```python
from build123d import *

# Parameters (mm, degrees)
SKETCH1_W           = 300
SKETCH1_H           = 80
BOSS_EXTRUDE1_DEPTH = 7
CHAMFER1_SIZE       = 15
CHAMFER1_SIZE2      = 25.980762114
CHAMFER3_SIZE       = 15
CHAMFER3_SIZE2      = 25.980762114
SKETCH2_R           = 11
CUT_EXTRUDE1_DEPTH  = 10
SKETCH3_R           = 11
SKETCH3_R_2         = 9.5
BOSS_EXTRUDE3_DEPTH = 0.8
CUT_EXTRUDE2_DEPTH  = 8
SKETCH5_R           = 15
CUT_EXTRUDE3_DEPTH  = 8
CUT_EXTRUDE4_DEPTH  = 8
SKETCH7_R           = 8
CUT_EXTRUDE6_DEPTH  = 8
SKETCH8_R           = 8
SKETCH8_R_2         = 7
BOSS_EXTRUDE4_DEPTH = 1.8
SKETCH9_R           = 1.5
CUT_EXTRUDE7_DEPTH  = 8
SKETCH10_R          = 12
CUT_EXTRUDE8_DEPTH  = 1
SKETCH11_R          = 1.5
CUT_EXTRUDE9_DEPTH  = 8
SKETCH12_R          = 2.6
SKETCH12_R_2        = 2.5
CUT_EXTRUDE10_DEPTH = 8
SKETCH13_R          = 4
CUT_EXTRUDE11_DEPTH = 4
SKETCH14_R          = 1.75
CUT_EXTRUDE12_DEPTH = 8
CUT_EXTRUDE13_DEPTH = 8
CUT_EXTRUDE14_DEPTH = 8
CUT_EXTRUDE15_DEPTH = 8
SKETCH18_R          = 3.25
CUT_EXTRUDE16_DEPTH = 4
CHAMFER4_SIZE       = 2
FILLET1_R           = 3
FILLET2_R           = 3
SKETCH19_R          = 2.6
CUT_EXTRUDE17_DEPTH = 8
SKETCH20_R          = 4.5
CUT_EXTRUDE18_DEPTH = 5
SKETCH21_W          = 9
SKETCH21_H          = 5
CUT_EXTRUDE19_DEPTH = 5
CHAMFER5_SIZE       = 5


with BuildPart() as part:
    # Sketch1 → Boss-Extrude1 (new body)
    with BuildSketch(Plane.XY):
        with Locations((150, 40)):
            Rectangle(SKETCH1_W, SKETCH1_H)
    extrude(amount=BOSS_EXTRUDE1_DEPTH)

    # Chamfer1
    chamfer1_edges = [part.edges().sort_by_distance(p)[0] for p in [
        (0, 0, 3.5),
    ]]
    chamfer1_side = [part.faces().sort_by_distance(p)[0] for p in [
        (0, 40, 3.5),
    ]]
    chamfer(chamfer1_edges, length=CHAMFER1_SIZE, length2=CHAMFER1_SIZE2, reference=chamfer1_side[0])

    # Chamfer3
    chamfer3_edges = [part.edges().sort_by_distance(p)[0] for p in [
        (0, 80, 3.5),
    ]]
    chamfer3_side = [part.faces().sort_by_distance(p)[0] for p in [
        (0, 47.5, 3.5),
    ]]
    chamfer(chamfer3_edges, length=CHAMFER3_SIZE, length2=CHAMFER3_SIZE2, reference=chamfer3_side[0])

    # Sketch2 → Cut-Extrude1 (cut)
    with BuildSketch(Plane.XY.offset(7)):
        with Locations((35, 40)):
            Circle(SKETCH2_R)
    extrude(amount=-CUT_EXTRUDE1_DEPTH, mode=Mode.SUBTRACT)

    # Sketch3 → Boss-Extrude3 (add)
    with BuildSketch(Plane.XY.offset(7)):
        with Locations((35, 40)):
            Circle(SKETCH3_R)
        with Locations((35, 40)):
            Circle(SKETCH3_R_2, mode=Mode.SUBTRACT)
    extrude(amount=-BOSS_EXTRUDE3_DEPTH)

    # Sketch4 → Cut-Extrude2 (cut, through all)
    with BuildSketch(Plane.XY.offset(7)):
        with BuildLine():
            Line((163.324941262, 70), (163.324941262, 40))
            ThreePointArc((163.324941262, 40), (162.324941262, 39), (161.324941262, 40))
            Line((161.324941262, 40), (161.324941262, 70))
            ThreePointArc((161.324941262, 70), (162.324941262, 71), (163.324941262, 70))
        make_face()
    extrude(amount=-CUT_EXTRUDE2_DEPTH, mode=Mode.SUBTRACT)

    # Sketch5 → Cut-Extrude3 (cut, through all)
    with BuildSketch(Plane.XY.offset(7)):
        with Locations((250, 40)):
            Circle(SKETCH5_R)
    extrude(amount=-CUT_EXTRUDE3_DEPTH, mode=Mode.SUBTRACT)

    # Sketch6 → Cut-Extrude4 (cut)
    with BuildSketch(Plane(origin=(0, 0, 0), x_dir=(-1, 0, 0), z_dir=(0, 0, -1))):
        with BuildLine():
            Line((-158.324941262, 70), (-158.324941262, 40))
            ThreePointArc((-158.324941262, 40), (-162.324941262, 36), (-166.324941262, 40))
            Line((-166.324941262, 40), (-166.324941262, 70))
            ThreePointArc((-166.324941262, 70), (-162.324941262, 74), (-158.324941262, 70))
        make_face()
    extrude(amount=-CUT_EXTRUDE4_DEPTH, mode=Mode.SUBTRACT)

    # Sketch7 → Cut-Extrude6 (cut, through all)
    with BuildSketch(Plane.XY.offset(7)):
        with Locations((113.691629607, 65)):
            Circle(SKETCH7_R)
    extrude(amount=-CUT_EXTRUDE6_DEPTH, mode=Mode.SUBTRACT)

    # Sketch8 → Boss-Extrude4 (add)
    with BuildSketch(Plane.XY.offset(7)):
        with Locations((113.691629607, 65)):
            Circle(SKETCH8_R)
        with Locations((113.691629607, 65)):
            Circle(SKETCH8_R_2, mode=Mode.SUBTRACT)
    extrude(amount=-BOSS_EXTRUDE4_DEPTH)

    # Sketch9 → Cut-Extrude7 (cut, through all)
    with BuildSketch(Plane(origin=(0, 0, 0), x_dir=(-1, 0, 0), z_dir=(0, 0, -1))):
        with Locations((-113.691629607, 74.75)):
            Circle(SKETCH9_R)
        with Locations((-105.24788192, 69.875)):
            Circle(SKETCH9_R)
        with Locations((-105.24788192, 60.125)):
            Circle(SKETCH9_R)
        with Locations((-113.691629607, 55.25)):
            Circle(SKETCH9_R)
        with Locations((-122.135377294, 60.125)):
            Circle(SKETCH9_R)
        with Locations((-122.135377294, 69.875)):
            Circle(SKETCH9_R)
    extrude(amount=-CUT_EXTRUDE7_DEPTH, mode=Mode.SUBTRACT)

    # Sketch10 → Cut-Extrude8 (cut)
    with BuildSketch(Plane(origin=(0, 0, 0), x_dir=(-1, 0, 0), z_dir=(0, 0, -1))):
        with Locations((-113.691629607, 65)):
            Circle(SKETCH10_R)
    extrude(amount=-CUT_EXTRUDE8_DEPTH, mode=Mode.SUBTRACT)

    # Sketch11 → Cut-Extrude9 (cut, through all)
    with BuildSketch(Plane(origin=(0, 0, 0), x_dir=(-1, 0, 0), z_dir=(0, 0, -1))):
        with Locations((-35, 52.875)):
            Circle(SKETCH11_R)
        with Locations((-23.849922926, 46.4375)):
            Circle(SKETCH11_R)
        with Locations((-23.849922926, 33.5625)):
            Circle(SKETCH11_R)
        with Locations((-35, 27.125)):
            Circle(SKETCH11_R)
        with Locations((-46.150077074, 33.5625)):
            Circle(SKETCH11_R)
        with Locations((-46.150077074, 46.4375)):
            Circle(SKETCH11_R)
    extrude(amount=-CUT_EXTRUDE9_DEPTH, mode=Mode.SUBTRACT)

    # Sketch12 → Cut-Extrude10 (cut, through all)
    with BuildSketch(Plane(origin=(0, 0, 0), x_dir=(-1, 0, 0), z_dir=(0, 0, -1))):
        with Locations((-35.980762114, 75)):
            Circle(SKETCH12_R)
        with Locations((-185.980762114, 75)):
            Circle(SKETCH12_R_2)
        with Locations((-295, 75)):
            Circle(SKETCH12_R_2)
        with Locations((-35.980762114, 5)):
            Circle(SKETCH12_R)
        with Locations((-185.980762114, 5)):
            Circle(SKETCH12_R_2)
        with Locations((-295, 5)):
            Circle(SKETCH12_R_2)
    extrude(amount=-CUT_EXTRUDE10_DEPTH, mode=Mode.SUBTRACT)

    # Sketch13 → Cut-Extrude11 (cut)
    with BuildSketch(Plane(origin=(0, 0, 0), x_dir=(-1, 0, 0), z_dir=(0, 0, -1))):
        with Locations((-295, 75)):
            Circle(SKETCH13_R)
        with Locations((-185.980762114, 75)):
            Circle(SKETCH13_R)
        with Locations((-35.980762114, 75)):
            Circle(SKETCH13_R)
        with Locations((-35.980762114, 5)):
            Circle(SKETCH13_R)
        with Locations((-185.980762114, 5)):
            Circle(SKETCH13_R)
        with Locations((-295, 5)):
            Circle(SKETCH13_R)
    extrude(amount=-CUT_EXTRUDE11_DEPTH, mode=Mode.SUBTRACT)

    # Sketch14 → Cut-Extrude12 (cut, through all)
    with BuildSketch(Plane.XY.offset(7)):
        with Locations((234.5, 55.5)):
            Circle(SKETCH14_R)
        with Locations((265.5, 55.5)):
            Circle(SKETCH14_R)
        with Locations((234.5, 24.5)):
            Circle(SKETCH14_R)
        with Locations((265.5, 24.5)):
            Circle(SKETCH14_R)
    extrude(amount=-CUT_EXTRUDE12_DEPTH, mode=Mode.SUBTRACT)

    # Sketch15 → Cut-Extrude13 (cut, through all)
    with BuildSketch(Plane.XY.offset(7)):
        Polygon((55.980762114, 0), (80.980762114, 25), (135.980762114, 25), (160.980762114, 0), align=None)
    extrude(amount=-CUT_EXTRUDE13_DEPTH, mode=Mode.SUBTRACT)

    # Sketch16 → Cut-Extrude14 (cut, through all)
    with BuildSketch(Plane.XY.offset(7)):
        Polygon((173.074478381, 25), (191.398328859, 61), (221.398328859, 61), (203.074478381, 25), align=None)
    extrude(amount=-CUT_EXTRUDE14_DEPTH, mode=Mode.SUBTRACT)

    # Sketch17 → Cut-Extrude15 (cut, through all)
    with BuildSketch(Plane.XY.offset(7)):
        with BuildLine():
            Line((129.537407736, 67.5), (150.148643313, 67.5))
            Line((150.148643313, 67.5), (150.148643313, 37.5))
            Line((150.148643313, 37.5), (62.386127875, 37.5))
            ThreePointArc((62.386127875, 37.5), (58.87799347, 53.641533192), (46.754644264, 64.861181352))
            Line((46.754644264, 64.861181352), (46.754644264, 67.5))
            Line((46.754644264, 67.5), (97.845851478, 67.5))
            ThreePointArc((97.845851478, 67.5), (113.691629607, 48.958220657), (129.537407736, 67.5))
        make_face()
    extrude(amount=-CUT_EXTRUDE15_DEPTH, mode=Mode.SUBTRACT)

    # Sketch18 → Cut-Extrude16 (cut)
    with BuildSketch(Plane.XY.offset(7)):
        with Locations((234.5, 55.5)):
            Circle(SKETCH18_R)
        with Locations((265.5, 55.5)):
            Circle(SKETCH18_R)
        with Locations((265.5, 24.5)):
            Circle(SKETCH18_R)
        with Locations((234.5, 24.5)):
            Circle(SKETCH18_R)
    extrude(amount=-CUT_EXTRUDE16_DEPTH, mode=Mode.SUBTRACT)

    # Chamfer4
    chamfer4_edges = [part.edges().sort_by_distance(p)[0] for p in [
        (235, 40, 7),
    ]]
    chamfer(chamfer4_edges, length=CHAMFER4_SIZE)

    # Fillet1
    fillet1_edges = [part.edges().sort_by_distance(p)[0] for p in [
        (203.074478381, 25, 3.5),
        (173.074478381, 25, 3.5),
        (191.398328859, 61, 3.5),
        (221.398328859, 61, 3.5),
    ]]
    fillet(fillet1_edges, radius=FILLET1_R)

    # Fillet2
    fillet2_edges = [part.edges().sort_by_distance(p)[0] for p in [
        (150.148643313, 67.5, 3.5),
        (150.148643313, 37.5, 3.5),
        (62.386127875, 37.5, 3.5),
    ]]
    fillet(fillet2_edges, radius=FILLET2_R)

    # Sketch19 → Cut-Extrude17 (cut, through all)
    with BuildSketch(Plane(origin=(0, 0, 0), x_dir=(-1, 0, 0), z_dir=(0, 0, -1))):
        with Locations((-280, 75)):
            Circle(SKETCH19_R)
        with Locations((-270, 75)):
            Circle(SKETCH19_R)
        with Locations((-270, 5)):
            Circle(SKETCH19_R)
        with Locations((-280, 5)):
            Circle(SKETCH19_R)
    extrude(amount=-CUT_EXTRUDE17_DEPTH, mode=Mode.SUBTRACT)

    # Sketch20 → Cut-Extrude18 (cut)
    with BuildSketch(Plane.XY.offset(7)):
        with Locations((270, 75)):
            Circle(SKETCH20_R)
        with Locations((280, 75)):
            Circle(SKETCH20_R)
        with Locations((280, 5)):
            Circle(SKETCH20_R)
        with Locations((270, 5)):
            Circle(SKETCH20_R)
    extrude(amount=-CUT_EXTRUDE18_DEPTH, mode=Mode.SUBTRACT)

    # Sketch21 → Cut-Extrude19 (cut)
    with BuildSketch(Plane.XY.offset(7)):
        with Locations((270, 77.5)):
            Rectangle(SKETCH21_W, SKETCH21_H)
        with Locations((280, 77.5)):
            Rectangle(SKETCH21_W, SKETCH21_H)
        with Locations((270, 2.5)):
            Rectangle(SKETCH21_W, SKETCH21_H)
        with Locations((280, 2.5)):
            Rectangle(SKETCH21_W, SKETCH21_H)
    extrude(amount=-CUT_EXTRUDE19_DEPTH, mode=Mode.SUBTRACT)

    # Chamfer5
    chamfer5_edges = [part.edges().sort_by_distance(p)[0] for p in [
        (275, 0, 7),
        (275, 80, 7),
    ]]
    chamfer(chamfer5_edges, length=CHAMFER5_SIZE)


solid = part.part
```
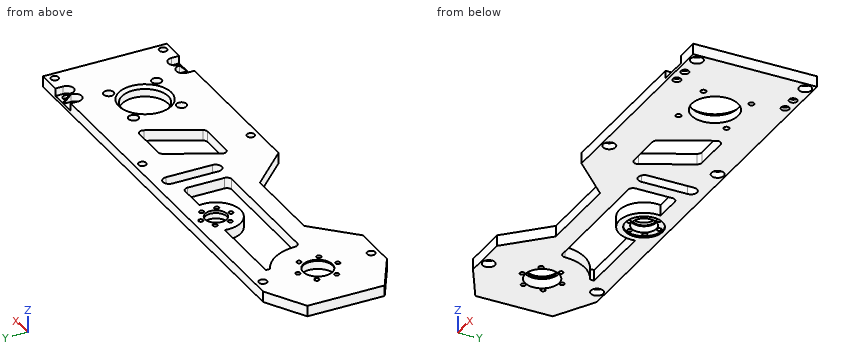
For this review, take the finished solid that the model builds, in its own axes (mm). Coordinates: 2 decimals unless noted, no trailing zeros. Loops run counter-clockwise (first coordinate to the right, second up) from the corner with the lowest first, then second, coordinate; pieces in that order, holes last. Notation, with made-up numbers: (71, 55.25) -> (80, 55.25) arc R17 ccw to (80, 84.25) -> close; hole circle Ø8 at (-11, 74). An arc over 180 degrees is marked (long way). Return JSON: item names as keys, results as strings. Group by question number.
(1) For pin 1 Ø5 at (x, y) = (95, 66.5) entering from +Z; pin 2 Ø4 at (y, z) = (78, 4.5) entering from -X; pin 3 Ø1.5 at (x, z) = (158.5, 4) entering from -Y; pin 4 Ø5 at (x, y) = (265, 55.5) entering from +Z, all flat-tipped, find the tip position at first contact; note any pin that passes through.
(2) Consider section A-A, the plane x = 139.5. Give the boundary of the cut face in (y, z), plus the area to 3 significant figures.
(3) To check wall thickness, follow L1, parallel to X at y = 36.5, z = 5.5; L2, parallel to X at y = 28, z = 5; L3, parallel to X at y = 34, z = 1.25. State the ranges of each line that lie inside material, in increasing order.
Results below:
{
 "1": {"pin 1": "stops at z = 7", "pin 2": "stops at x = 19.05", "pin 3": "stops at y = 1.73", "pin 4": "stops at z = 3"},
 "2": {"outline": "(21.48, 0) -> (37.5, 0) -> (37.5, 7) -> (21.48, 7) -> close; (67.5, 0) -> (80, 0) -> (80, 7) -> (67.5, 7) -> close", "area": "200 mm2"},
 "3": {"L1": "x = 0 to 24.57, 45.43 to 160.39, 164.26 to 178.93, 208.93 to 234.9, 265.1 to 300", "L2": "x = 0 to 33.78, 36.22 to 174.97, 204.6 to 241, 259 to 300", "L3": "x = 0 to 22.42, 25.28 to 25.78, 44.22 to 44.72, 47.58 to 177.66, 207.66 to 236.25, 263.75 to 300"}
}
